The model under review builds one solid part; all positions refer to its coordinate system, in mm. A direction names the side the tool comes from. Coordinates: 2 decimals unless noted, no trailing zeros. Loops run counter-clockwise (first coordinate to the right, second up) from the corner with the lowest first, then second, coordinate; pieces in that order, holes last. Notation, with made-up numbers: (30, -28) - (52, -28) arc R22 ccw to (52, 8) - close; hole circle Ø10 at (-8.75, -38.5). An arc over 180 degrees is marked (long way). One line per item, written item: value. Start each with the question number.
1. We need section D-D, the plane z = -5. Give the boundary of the cut face in (x, y) (1 decimal).
2. We need section B-B, the plane z = 0. Give the boundary of the cut face in (x, y) (1 decimal).
3. We need section C-C, the plane x = 18. Give the boundary of the cut face in (y, z) (3 decimals), then the cut area to 3 significant figures.
4. To check wall thickness, follow line 1 (X direction, y = 4.5, z = 0) (3 decimals); line 2 (Z direction, x = -13.5, y = 17); line 3 (Y direction, x = 10.5, z = 19). State the ranges of each line that lie inside material, in increasing order.
5. Insertion check: P1, Ø19, axis at x = -14.5, z = 2.5, coming from the +Y side. The pin has a flat end and moves straight along its axis. Give the tip position at first contact, or say it passes through.
6. Mouldability with a two-part tool opening along Z and no side actions: class faces 1 (the face through (11.53, 6.44, 0.26)), 2 (the face through (0, 6, 22.225)), 3 (the face through (13, 22.86, -14)), 4 (the face through (0, 6, -22.225)) as +Z half, -Z half, draft (parallel to the pull), parting line (faces both ways), or undercut.
7. We need section A-A, the plane y = 9.5. Give the boundary of the cut face in (x, z) (3 decimals), then the cut area to 3 significant figures.
8. For faces 5 (the face through (-11.07, 16.93, -12.73)), 6 (the face through (-0.1, 7.94, 0.31)), list the 3-axis set-ups (+Z, -Z, +X, -X, +Y, -Y) from which the entire face can be reached by the end or side of a thin tool; tool diameter is ignored.
Autodesk Inventor part; units mm, degrees
ref_plane "YZ Plane" through (0, 0, 0) normal (1, 0, 0) x (0, 1, 0)
ref_plane "XZ Plane" through (0, 0, 0) normal (0, 1, 0) x (-1, 0, 0)
ref_plane "XY Plane" through (0, 0, 0) normal (0, 0, 1) x (1, 0, 0)
sketch "Sketch1" plane through (0, 0, 0) normal (0, 1, 0) x (-1, 0, 0)
  line L0 (-22.225, 22.225) -> (-22.225, -22.225)
  line L1 (-22.225, -22.225) -> (22.225, -22.225)
  line L2 (22.225, -22.225) -> (22.225, 22.225)
  line L3 (22.225, 22.225) -> (-22.225, 22.225)
  line L4 (-22.225, 22.225) -> (22.225, -22.225) construction
  line L5 (-22.225, -22.225) -> (22.225, 22.225) construction
  point P0 (0, 0)
  dimension "d0" = 44.45
extrude "Extrusion1" add sketch "Sketch1" along normal blind 12.7
sketch "Sketch2" plane through (-22.225, 0, 22.225) normal (0, 0, 1) x (1, 0, 0)
  line L0 (44.45, 12.7) -> (0, 12.7)
  arc A0 (17.4625, 12.7) -> (26.9875, 12.7) centre (22.225, 12.7) ccw
  point P0 (22.225, 0)
  dimension "d3" = 9.525
extrude "Extrusion2" cut sketch "Sketch2" against normal through all
sketch "Sketch3" plane through (0, 0, 0) normal (0, -1, 0) x (1, 0, 0)
  line L0 (-22.225, -22.225) -> (-22.225, 22.225)
  line L1 (22.225, 22.225) -> (22.225, -22.225)
  line L2 (-22.225, 22.225) -> (-4.7625, 22.225)
  line L3 (4.7625, 22.225) -> (22.225, 22.225)
  point P0 (0, 0)
  point P1 (-13.4938, 0)
  point P2 (13.4938, 0)
  dimension "d6" = 8.7312
  dimension "d7" = 8.7312
  dimension "d22" = 22.225
  dimension "d23" = 22.225
hole "Hole1" at (-13.4938, 0, 0) at (13.4938, 0, 0) direction (0, 1, 0) diameter 3.9624 end through all
sketch "Sketch7" plane through (0, 12.7, 0) normal (0, 1, 0) x (1, 0, 0)
  line L0 (-13.4938, -13.4938) -> (13.4938, -13.4938) construction
  line L1 (13.4938, -13.4938) -> (13.4938, 13.4938) construction
  line L2 (13.4938, 13.4938) -> (-13.4938, 13.4938) construction
  line L3 (-13.4938, 13.4938) -> (-13.4938, -13.4938) construction
  line L4 (-13.4938, -13.4938) -> (13.4938, 13.4938) construction
  line L5 (13.4938, -13.4938) -> (-13.4938, 13.4938) construction
  line L6 (-22.225, 22.225) -> (-22.225, -22.225) construction
  line L7 (-22.225, -22.225) -> (-4.7625, -22.225) construction
  circle A0 centre (-13.4938, -13.4938) radius 2.54
  circle A1 centre (-13.4938, 13.4938) radius 2.54
  circle A2 centre (13.4938, 13.4938) radius 2.54
  circle A3 centre (13.4938, -13.4938) radius 2.54
  point P0 (0, 0)
  dimension "d26" = 8.7312
  dimension "d27" = 8.7312
  dimension "d28" = 5.08
extrude "Extrusion3" add sketch "Sketch7" along normal blind 10.16
fillet "Fillet1" radius 1.5875 4 edges at (-16.0338, 22.86, 13.4938) (-16.0338, 22.86, -13.4938) (10.9537, 22.86, -13.4938) (10.9537, 22.86, 13.4938)
sketch "Sketch4" plane through (0, 12.7, 0) normal (0, 1, 0) x (1, 0, 0)
  point P0 (-11.9062, 0)
equation "\"d0\" = baseWidth"
equation "\"d1\" = heightOfBottomSupport"
equation "\"d3\" = bottomHoleDiam"
equation "\"d4\" = deltaBottomToTop"
equation "\"d26\" = edgeToBoltHole"
equation "\"d27\" = edgeToBoltHole"
equation "\"d28\" = supportHoleDiam"
equation "\"d29\" = supportHoleLength"
equation "\"bottomHoleDiam\" = 9.525"
equation "\"baseWidth\" = 44.45"
equation "\"height\" = deltaBottomToTop + heightOfBottomHole + heightOfTopHole"
equation "\"deltaBottomToTop\" = 25.4"
equation "\"topHoleDiam\" = 9.525"
equation "\"edgeToBoltHole\" = -0.25 * bottomHoleDiam + 0.25 * baseWidth"
equation "\"washerDiam\" = 13.97"
equation "\"depthForSocketHead\" = 6.35"
equation "\"xbottomHoleDiam\" = 9.525"
equation "\"baseLength\" = 38.1"
equation "\"heightOfBottomSupport\" = 12.7"
equation "\"supportHoleDiam\" = 5.08"
equation "\"supportHoleLength\" = 10.16"
properties part number "BottomOfSquareSupport" material "PC/ABS Plastic"
Findings below:
1. outline: (-22.2, 0) - (22.2, 0) - (22.2, 12.7) - (4.8, 12.7) arc R4.8 cw to (-4.8, 12.7) - (-22.2, 12.7) - close
2. outline: (-22.2, 0) - (-15.5, 0) - (-15.5, 12.7) - (-22.2, 12.7) - close; (-11.5, 0) - (11.5, 0) - (11.5, 12.7) - (4.8, 12.7) arc R4.8 cw to (-4.8, 12.7) - (-11.5, 12.7) - close; (15.5, 0) - (22.2, 0) - (22.2, 12.7) - (15.5, 12.7) - close
3. outline: (0, -22.225) - (12.7, -22.225) - (12.7, 22.225) - (0, 22.225) - close
3. area: 565 mm2
4. line 1: -22.225 to -15.475, -11.513 to 11.513, 15.475 to 22.225
4. line 2: -16.03 to -10.95, 10.95 to 16.03
4. line 3: 0 to 12.7
5. P1: y = 22.75
6. face 1: undercut
6. face 2: +Z half
6. face 3: draft
6. face 4: -Z half
7. outline: (-22.225, -22.225) - (-3.527, -22.225) - (-3.527, 22.225) - (-22.225, 22.225) - close; (3.527, -22.225) - (22.225, -22.225) - (22.225, 22.225) - (3.527, 22.225) - close; hole circle Ø3.962 at (-13.494, 0); hole circle Ø3.962 at (13.494, 0)
7. area: 1,640 mm2
8. face 5: +Y
8. face 6: +Z, -Z, +Y
